Can you work these out from the model? Positions are in its coordinate system, mm. A direction names the side the tool comes from. Coordinates: 2 decimals unless noted, no trailing zeros. Write each loop counter-clockwise with the first axis right and the second up, starting at its lowest first coordinate (ties: lowest second). Pieces come first, ordered by that corner, then holes. Notation, with made-up numbers: (-14, 46) - (-3, 46) arc R18 ccw to (-3, 52) - close; hole circle Ø10 at (60.5, 23.5). An arc over 180 degrees is marked (long way). Write each question's results on one line, items separated by ' | '. Start each with the question number.
```python
from build123d import *

# Parameters (mm, degrees)
SKETCH1_R               = 12
BOSS_EXTRUDE1_DEPTH     = 12.5
SKETCH2_R               = 4
BOSS_EXTRUDE2_DEPTH     = 4.5
SHELL1_T                = -1.5
CHAMFER2_SIZE           = 1
SKETCH3_R               = 6
SKETCH3_R_2             = 4
BOSS_EXTRUDE3_DEPTH     = 0.5
BOSS_EXTRUDE4_DEPTH     = 11
MIRROR2_COPY_1_DEPTH    = 11
SKETCH5_R               = 1.5
BOSS_EXTRUDE5_DEPTH     = 11
MIRROR4_COPY_1_SKETCH_R = 1.5
MIRROR4_COPY_1_DEPTH    = 11
SKETCH6_R               = 0.75
CUT_EXTRUDE1_DEPTH      = 8
MIRROR6_COPY_1_SKETCH_R = 0.75
MIRROR6_COPY_1_DEPTH    = 8


with BuildPart() as part:
    # Sketch1 → Boss-Extrude1 (new body)
    with BuildSketch(Plane(origin=(0, 0, 0), x_dir=(1, 0, 0), z_dir=(0, 1, 0))):
        with Locations(Location((0, 0, 0), (0, 0, 270))):
            Circle(SKETCH1_R)
    extrude(amount=BOSS_EXTRUDE1_DEPTH)

    # Sketch2 → Boss-Extrude2 (add)
    with BuildSketch(Plane(origin=(0, 12.5, 0), x_dir=(1, 0, 0), z_dir=(0, 1, 0))):
        with Locations(Location((0, 0, 0), (0, 0, 270))):
            Circle(SKETCH2_R)
    extrude(amount=BOSS_EXTRUDE2_DEPTH)

    # Shell1
    shell1_openings = [part.faces().sort_by_distance(p)[0] for p in [
        (0, 0, 0),
        (0, 17, 0),
    ]]
    offset(amount=SHELL1_T, openings=shell1_openings, kind=Kind.INTERSECTION)

    # Chamfer2
    chamfer2_edges = [part.edges().sort_by_distance(p)[0] for p in [
        (0, 12.5, -12),
    ]]
    chamfer(chamfer2_edges, length=CHAMFER2_SIZE)

    # Sketch3 → Boss-Extrude3 (add)
    with BuildSketch(Plane(origin=(0, 12.5, 0), x_dir=(1, 0, 0), z_dir=(0, 1, 0))):
        with Locations(Location((0, 0, 0), (0, 0, 270))):
            Circle(SKETCH3_R)
        with Locations(Location((0, 0, 0), (0, 0, 270))):
            Circle(SKETCH3_R_2, mode=Mode.SUBTRACT)
    extrude(amount=BOSS_EXTRUDE3_DEPTH)

    # Sketch4 → Boss-Extrude4 (add)
    with BuildSketch(Plane(origin=(0, 0, 0), x_dir=(1, 0, 0), z_dir=(0, 1, 0))):
        with BuildLine():
            Line((-2.5, -10.198039027), (-2.5, -8.392304845))
            Line((-2.5, -8.392304845), (-1.5, -8.392304845))
            Line((-1.5, -8.392304845), (-1.5, -10.392304845))
            ThreePointArc((-1.5, -10.392304845), (-2.002357311, -10.307306399), (-2.5, -10.198039027))
        make_face()
    boss_extrude4 = extrude(amount=BOSS_EXTRUDE4_DEPTH)

    # Mirror1: Boss-Extrude4 across plane
    add(boss_extrude4.mirror(Plane(origin=(0, 0, 0), x_dir=(0, 0, 1), z_dir=(1, 0, 0))))

    # Mirror2: Boss-Extrude4 across plane
    add(boss_extrude4.mirror(Plane.XY))

    # Mirror2 copy 1 sketch → Mirror2 copy 1 (add)
    with BuildSketch(Plane(origin=(0, 0, 0), x_dir=(-1, 0, 0), z_dir=(0, 1, 0))):
        with BuildLine():
            Line((-2.5, -10.198039027), (-2.5, -8.392304845))
            Line((-2.5, -8.392304845), (-1.5, -8.392304845))
            Line((-1.5, -8.392304845), (-1.5, -10.392304845))
            ThreePointArc((-1.5, -10.392304845), (-2.002357311, -10.307306399), (-2.5, -10.198039027))
        make_face()
    extrude(amount=MIRROR2_COPY_1_DEPTH)

    # Sketch5 → Boss-Extrude5 (add)
    with BuildSketch(Plane(origin=(0, 0, 0), x_dir=(1, 0, 0), z_dir=(0, 1, 0))):
        with Locations((-8.25, -6.495190528)):
            Circle(SKETCH5_R)
    boss_extrude5 = extrude(amount=BOSS_EXTRUDE5_DEPTH)

    # Mirror3: Boss-Extrude5 across plane
    add(boss_extrude5.mirror(Plane(origin=(0, 0, 0), x_dir=(0, 0, 1), z_dir=(1, 0, 0))))

    # Mirror4: Boss-Extrude5 across plane
    add(boss_extrude5.mirror(Plane.XY))

    # Mirror4 copy 1 sketch → Mirror4 copy 1 (add)
    with BuildSketch(Plane(origin=(0, 0, 0), x_dir=(-1, 0, 0), z_dir=(0, 1, 0))):
        with Locations((-8.25, -6.495190528)):
            Circle(MIRROR4_COPY_1_SKETCH_R)
    extrude(amount=MIRROR4_COPY_1_DEPTH)

    # Sketch6 → Cut-Extrude1 (cut)
    with BuildSketch(Plane(origin=(0, 0, 0), x_dir=(1, 0, 0), z_dir=(0, 1, 0))):
        with Locations(Location((-8.25, -6.495190528, 0), (0, 0, 270))):
            Circle(SKETCH6_R)
    cut_extrude1 = extrude(amount=CUT_EXTRUDE1_DEPTH, mode=Mode.SUBTRACT)

    # Mirror5: Cut-Extrude1 across plane
    add(cut_extrude1.mirror(Plane(origin=(0, 0, 0), x_dir=(0, 0, 1), z_dir=(1, 0, 0))), mode=Mode.SUBTRACT)

    # Mirror6: Cut-Extrude1 across plane
    add(cut_extrude1.mirror(Plane.XY), mode=Mode.SUBTRACT)

    # Mirror6 copy 1 sketch → Mirror6 copy 1 (cut)
    with BuildSketch(Plane(origin=(0, 0, 0), x_dir=(-1, 0, 0), z_dir=(0, 1, 0))):
        with Locations(Location((-8.25, -6.495190528, 0), (0, 0, 270))):
            Circle(MIRROR6_COPY_1_SKETCH_R)
    extrude(amount=MIRROR6_COPY_1_DEPTH, mode=Mode.SUBTRACT)


solid = part.part
```
Q1. If we section it at A-A (x = 0): Please give me the cut outline in (y, z), then the cut area to 3 significant figures.
Q2. I'm going to push flat-ended pins straight in: pin 1 Ø6 at (y, z) = (10, 7.5) entering from -X; pin 2 Ø1.6 at (x, z) = (8.5, -6.5) entering from -Y; pin 3 Ø0.9 at (x, z) = (8.25, 6.5) entering from +Y; pin 4 Ø0.5 at (x, y) = (2, 3.5) entering from -Z. Where does each tip first touch, or does it pass through?
Q3. I need wall thicknesses on line 1 along X through (y, z) = (6.5, 7); line 2 along Z through (x, y) = (8.25, 6.25); line 3 along X through (y, z) = (15.75, 0). Which ranges of each line are inside material? Lowest first, please. Write a range as from..to.
Q4. If we section it at B-B (z = 0): Please give me the cut outline in (x, y).
Q5. Thinking about a two-plate mould opening in X: for faces 4 (the face through (2, 0, -9)), 5 (the face through (3.604, 5.67, 11.446)), 6 (the face through (-2, 5, 8.392)), which applies, pulls with the +X half, pulls with the -X half, needs draft (parallel to the pull), parting line crosses it, or undercut?
Q6. If we section it at C-C (y = 3.5): Count the separate pieces of the cut face and the enclosed holes in it, then the cut area to 3 significant figures.
Q7. For faces 1 (the face through (-3.905, 14.972, -0.867)), 2 (the face through (-2.44, 13.96, -0.54)), 3 (the face through (1.5, 5, -9)), which set-ups out of +Z, -Z, +X, -X, +Y, -Y let a thin tool reach every point of the face, with its end or its side?
Answer list:
1) outline: (0, -12) - (11.5, -12) - (12.5, -11) - (12.5, -6) - (13, -6) - (13, -4) - (17, -4) - (17, -2.5) - (11, -2.5) - (11, -10.5) - (0, -10.5) - close; (0, 10.5) - (11, 10.5) - (11, 2.5) - (17, 2.5) - (17, 4) - (13, 4) - (13, 6) - (12.5, 6) - (12.5, 11) - (11.5, 12) - (0, 12) - close | area: 76.0 mm2
2) pin 1: stops at x = -11.12 | pin 2: stops at y = 0 | pin 3: stops at y = 12.5 | pin 4: stops at z = -11.87
3) line 1: x = -9.75..-8.8, -7.7..-6.84, 6.84..7.7, 8.8..9.75 | line 2: z = -8.71..-7.25, -5.75..-5, 5..5.75, 7.25..8.71 | line 3: x = -4..-2.5, 2.5..4
4) outline: (-12, 0) - (-10.5, 0) - (-10.5, 11) - (-2.5, 11) - (-2.5, 17) - (-4, 17) - (-4, 13) - (-6, 13) - (-6, 12.5) - (-11, 12.5) - (-12, 11.5) - close; (2.5, 11) - (10.5, 11) - (10.5, 0) - (12, 0) - (12, 11.5) - (11, 12.5) - (6, 12.5) - (6, 13) - (4, 13) - (4, 17) - (2.5, 17) - close
5) face 4: needs draft | face 5: parting line crosses it | face 6: undercut
6) separate pieces: 1 | enclosed holes: 5 | area: 120 mm2
7) face 1: +Y | face 2: +Y, -Y | face 3: -Y
